```python
from build123d import *

# Parameters (mm, degrees)
SKETCH054_R     = 48
SKETCH054_R_2   = 38.75
PAD029_DEPTH    = 1.6
PAD030_DEPTH    = 1
FILLET018_R     = 0.8
POCKET029_DEPTH = 5
FILLET020_R     = 1


with BuildPart() as part:
    # Sketch054 → Pad029 (new body)
    with BuildSketch(Plane.XY):
        Circle(SKETCH054_R)
        Circle(SKETCH054_R_2, mode=Mode.SUBTRACT)
    extrude(amount=PAD029_DEPTH)

    # Sketch055 → Pad030 (join)
    with BuildSketch(Plane(origin=(0, 0, 0), x_dir=(-1, 0, 0), z_dir=(0, 0, -1))):
        with BuildLine():
            ThreePointArc((-1.3, 46.94), (-2.2, 46.04), (-1.3, 45.14))
            Line((-1.3, 45.14), (1.3, 45.14))
            ThreePointArc((1.3, 45.14), (2.2, 46.04), (1.3, 46.94))
            Line((1.3, 46.94), (-1.3, 46.94))
        make_face()
        with BuildLine():
            ThreePointArc((-1.3, 44.4), (-2.2, 43.5), (-1.3, 42.6))
            Line((-1.3, 42.6), (1.3, 42.6))
            ThreePointArc((1.3, 42.6), (2.2, 43.5), (1.3, 44.4))
            Line((1.3, 44.4), (-1.3, 44.4))
        make_face()
        with BuildLine():
            ThreePointArc((-1.3, 41.86), (-2.2, 40.96), (-1.3, 40.06))
            Line((-1.3, 40.06), (1.3, 40.06))
            ThreePointArc((1.3, 40.06), (2.2, 40.96), (1.3, 41.86))
            Line((1.3, 41.86), (-1.3, 41.86))
        make_face()
        with BuildLine():
            ThreePointArc((-13.374691, 45.088405), (-14.042506, 44.004882), (-12.958983, 43.337066))
            Line((-12.958983, 43.337066), (-10.429272, 43.937534))
            ThreePointArc((-10.429272, 43.937534), (-9.761456, 45.021057), (-10.84498, 45.688872))
            Line((-10.84498, 45.688872), (-13.374691, 45.088405))
        make_face()
        with BuildLine():
            ThreePointArc((-12.788343, 42.618178), (-13.456159, 41.534655), (-12.372635, 40.86684))
            Line((-12.372635, 40.86684), (-9.842924, 41.467307))
            ThreePointArc((-9.842924, 41.467307), (-9.175109, 42.55083), (-10.258632, 43.218646))
            Line((-10.258632, 43.218646), (-12.788343, 42.618178))
        make_face()
        with BuildLine():
            ThreePointArc((-12.201996, 40.147952), (-12.869811, 39.064428), (-11.786288, 38.396613))
            Line((-11.786288, 38.396613), (-9.256577, 38.99708))
            ThreePointArc((-9.256577, 38.99708), (-8.588761, 40.080604), (-9.672285, 40.748419))
            Line((-9.672285, 40.748419), (-12.201996, 40.147952))
        make_face()
    extrude(amount=PAD030_DEPTH)

    # Fillet018
    fillet018_edges = [part.edges().sort_by_distance(p)[0] for p in [
        (9.761456, 45.021057, -1),
        (9.175109, 42.55083, -1),
        (8.588761, 40.080604, -1),
        (-2.2, 40.96, -1),
        (-2.2, 43.5, -1),
        (-2.2, 46.04, -1),
    ]]
    fillet(fillet018_edges, radius=FILLET018_R)

    # Sketch060 → Pocket029 (cut)
    with BuildSketch(Plane.XY):
        with BuildLine():
            ThreePointArc((7.655731, 37.986212), (6.919079, 38.127272), (6.179836, 38.254047))
            Line((6.179836, 38.254047), (7.149736, 39.398292))
            Line((7.149736, 39.398292), (7.655731, 37.986212))
        make_face()
    extrude(amount=POCKET029_DEPTH, mode=Mode.SUBTRACT)

    # Fillet020
    fillet020_edges = [part.edges().sort_by_distance(p)[0] for p in [
        (7.655731, 37.986212, 0.8),
        (6.179836, 38.254047, 0.8),
    ]]
    fillet(fillet020_edges, radius=FILLET020_R)


solid = part.part
```
Verification items for the finished model (mm, model axes). Coordinates: 2 decimals unless noted, no trailing zeros. Loops run counter-clockwise (first coordinate to the right, second up) from the corner with the lowest first, then second, coordinate; pieces in that order, holes last. Notation, with made-up numbers: (25.5, 12) - (52.5, 12) arc R19 cw to (52.5, 29) - close; hole circle Ø6 at (54.25, 73). An arc over 180 degrees is marked (long way). Return JSON: item names as keys, results as strings.
1. Go/stop test with flat-tipped pins: pin 1 (1.5 mm diameter, centred on x = 15.5, z = 0, fed in from -Y); pin 2 (1.5 mm diameter, centred on x = -21, y = -38, fed in from -Z); pin 3 (3 mm diameter, centred on x = -33, y = 20, fed in from +Z). Record where each tip stops, or that it passes through.
Established:
{"pin 1": "stops at y = -45.68", "pin 2": "stops at z = 0", "pin 3": "stops at z = 1.6"}
2. Section check B-B, the plane y = 9.5. Record the boundary of the cut face in (x, z), then the cut area to 3 significant figures.
Established:
{"outline": "(-47.05, 0) - (-37.57, 0) - (-37.57, 1.6) - (-47.05, 1.6) - close; (37.57, 0) - (47.05, 0) - (47.05, 1.6) - (37.57, 1.6) - close", "area": "30.3 mm2"}
3. Thickness scan on L1, parallel to Y at x = 0, z = 1.1; L2, parallel to Y at x = 11, z = -0.05; L3, parallel to Y at x = 26.5, z = 0.4. Record the ranges inside material, lowest first.
Established:
{"L1": "y = -48 to -38.75, 38.75 to 48", "L2": "y = 38.58 to 40.43, 41.19 to 43.04, 43.8 to 45.65", "L3": "y = -40.02 to -28.27, 28.27 to 40.02"}
4. Section check D-D, the plane y = -40.5. Record the boundary of the cut face in (x, z), then the cut area to 3 significant figures.
Established:
{"outline": "(-25.76, 0) - (25.76, 0) - (25.76, 1.6) - (-25.76, 1.6) - close", "area": "82.4 mm2"}
5. Section check A-A, the plane x = 4. Record the boundary of the cut face in (y, z), then the cut area to 3 significant figures.
Established:
{"outline": "(-47.83, 0) - (-38.54, 0) - (-38.54, 1.6) - (-47.83, 1.6) - close; (38.54, 0) - (47.83, 0) - (47.83, 1.6) - (38.54, 1.6) - close", "area": "29.7 mm2"}
6. Section check C-C, the plane z = 1. Record the boundary of the cut face in (x, y), then the cut area to 3 significant figures.
Established:
{"outline": "circle Ø96 at (0, 0); hole (5.63, 38.34) arc R38.75 ccw (long way) to (8.2, 37.87) arc R1 cw to (7.47, 38.51) - (7.15, 39.4) - (6.54, 38.68) arc R1 cw to start", "area": "2,520 mm2"}
